from build123d import *

# Parameters (mm, degrees)
F0_R     = 6
F1_DEPTH = 1
F2_R     = 5
F3_DEPTH = 6
F5_DEPTH = 6
F6_R     = 0.2
F7_R     = 0.1


with BuildPart() as f1:
    # F0 (on Front) → F1 (new body)
    with BuildSketch(Plane.XZ):
        Circle(F0_R)
    extrude(amount=-F1_DEPTH)

    # F2 (on face) → F3 (join)
    with BuildSketch(Plane.XZ):
        Circle(F2_R)
    extrude(amount=F3_DEPTH)

    # F4 (on face) → F5 (cut)
    with BuildSketch(Plane.XZ.offset(6)):
        Polygon((3.6786964709, 0.7419741291), (1.1967797907, 3.5568316612), (-2.4819166802, 2.8148575321), (-3.6786964709, -0.7419741291), (-1.1967797907, -3.5568316612), (2.4819166802, -2.8148575321), align=None)
    extrude(amount=-F5_DEPTH, mode=Mode.SUBTRACT)

    # F6
    f6_edges = [f1.edges().sort_by_distance(p)[0] for p in [
        (-5, -6, 0),
        (0.642568, -6, -3.185845),
        (3.080307, -6, -1.036442),
        (2.437738, -6, 2.149403),
        (-0.642568, -6, 3.185845),
        (-3.080307, -6, 1.036442),
        (-2.437738, -6, -2.149403),
    ]]
    fillet(f6_edges, radius=F6_R)

    # F7
    f7_edges = [f1.edges().sort_by_distance(p)[0] for p in [
        (-6, 0, 0),
    ]]
    fillet(f7_edges, radius=F7_R)


solid = f1.part
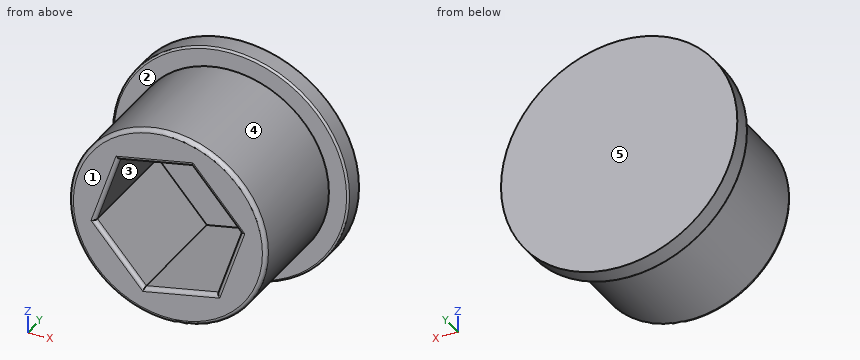
Verification items for the finished model (mm, model axes). Face numbers are marked on the shaded views. A direction names the side the tool comes from. Round coordinates to 2 decimals unless told otherwise and drop trailing zeros. Order: outer loops, then holes, each group sorted by start corner. A loop starts at its lowest first (then second) coordinate and runs counter-clockwise, first axis right, second up.
1. Thickness scan on L1, parallel to Y at x = -1, z = -1.25; L2, parallel to X at y = -2.5, z = 2.5; L3, parallel to X at y = -5.25, z = 1.5. Record the ranges inside material, lowest first.
Final values:
L1: y = 0 to 1
L2: x = -4.33 to -2.59, 2.13 to 4.33
L3: x = -4.77 to -2.92, 3.01 to 4.77
2. Access from +Z, -Z, +X, -X, +Y, -Y to the whole of each face (thin tool, end or side, straight path). Record for the marked faces 1 and 2.
Final values:
face 1: +Z, -Z, +X, -X, -Y
face 2: -Y
3. Release check for a two-part mould opening along X. For the marked faces 3, 4 and 5 record: +X half, -X half, draft (parallel to the pull), parting line (faces both ways), or undercut.
Final values:
face 3: undercut
face 4: parting line
face 5: draft
4. Go/stop test with a flat-tipped pin: P1, Ø2, axis at x = 4, y = -2, coming from the +Z side. Record where the tip stops, or that it passes through.
Final values:
P1: stops at z = 4
5. Section check A-A on y = -5. Record the cut outline in (x, z), then the cut area to 3 significant figures.
Final values:
outline: circle Ø10 at (0, 0); hole (-3.68, -0.74) - (-1.2, -3.56) - (2.48, -2.81) - (3.68, 0.74) - (1.2, 3.56) - (-2.48, 2.81) - close
area: 42.0 mm2
